```python
from build123d import *

# Parameters (mm, degrees)
SKETCH1_W            = 59.589999946
SKETCH1_H            = 23.283333334
BOSS_EXTRUDE1_DEPTH  = 2.929999982
SKETCH2_W            = 2.929999982
SKETCH2_H            = 11.641666667
CUT_EXTRUDE1_DEPTH   = 3.929999982
BOSS_EXTRUDE3_DEPTH  = 2.93
FILLET1_R            = 0.2
SKETCH5_R            = 0.25
CUT_EXTRUDE3_DEPTH   = 3.93
FILLET2_R            = 0.5
FILLET1_OF_MIRROR1_R = 0.2
FILLET2_OF_MIRROR1_R = 0.5
SKETCH3_W            = 44.45
SKETCH3_H            = 16.933333334
CUT_EXTRUDE2_DEPTH   = 1


with BuildPart() as part:
    # Sketch1 → Boss-Extrude1 (new body)
    with BuildSketch(Plane.XY):
        Rectangle(SKETCH1_W, SKETCH1_H)
    extrude(amount=BOSS_EXTRUDE1_DEPTH)

    # Sketch2 → Cut-Extrude1 (cut, through all)
    with BuildSketch(Plane.XY.offset(2.929999982)):
        with Locations((-26.864999991, -5.820833334)):
            Rectangle(SKETCH2_W, SKETCH2_H)
    cut_extrude1 = extrude(amount=-CUT_EXTRUDE1_DEPTH, mode=Mode.SUBTRACT)

    # Sketch4 → Boss-Extrude3 (add)
    with BuildSketch(Plane.XY.offset(2.929999982)):
        Polygon((-27.329999982, -8.711666685), (-28.329999982, -8.711666685), (-28.329999982, -10.711666685), (-27.329999982, -9.711666685), align=None)
    boss_extrude3 = extrude(amount=-BOSS_EXTRUDE3_DEPTH)

    # Fillet1
    fillet1_edges = [part.edges().sort_by_distance(p)[0] for p in [
        (-27.329999982, -8.711666685, 1.464999982),
        (-28.329999982, -10.711666685, 1.464999982),
        (-27.329999982, -9.711666685, 1.464999982),
    ]]
    fillet(fillet1_edges, radius=FILLET1_R)

    # Sketch5 → Cut-Extrude3 (cut, through all)
    with BuildSketch(Plane.XY.offset(2.929999982)):
        with Locations((-28.329999982, 0)):
            Circle(SKETCH5_R)
    cut_extrude3 = extrude(amount=-CUT_EXTRUDE3_DEPTH, mode=Mode.SUBTRACT)

    # Fillet2
    fillet2_edges = [part.edges().sort_by_distance(p)[0] for p in [
        (-28.079999982, 0, 1.464999991),
        (-28.329999982, -0.25, 1.464999991),
    ]]
    fillet(fillet2_edges, radius=FILLET2_R)

    # Mirror1: Cut-Extrude1, Boss-Extrude3, Cut-Extrude3 across plane
    add(cut_extrude1.mirror(Plane(origin=(0, 0, 0), x_dir=(0, 0, 1), z_dir=(1, 0, 0))), mode=Mode.SUBTRACT)
    add(boss_extrude3.mirror(Plane(origin=(0, 0, 0), x_dir=(0, 0, 1), z_dir=(1, 0, 0))))
    add(cut_extrude3.mirror(Plane(origin=(0, 0, 0), x_dir=(0, 0, 1), z_dir=(1, 0, 0))), mode=Mode.SUBTRACT)

    # Fillet1 of Mirror1
    fillet1_of_mirror1_edges = [part.edges().sort_by_distance(p)[0] for p in [
        (27.329999982, -8.711666685, 1.464999982),
        (28.329999982, -10.711666685, 1.464999982),
        (27.329999982, -9.711666685, 1.464999982),
    ]]
    fillet(fillet1_of_mirror1_edges, radius=FILLET1_OF_MIRROR1_R)

    # Fillet2 of Mirror1
    fillet2_of_mirror1_edges = [part.edges().sort_by_distance(p)[0] for p in [
        (28.079999982, 0, 1.464999991),
        (28.329999982, -0.25, 1.464999991),
    ]]
    fillet(fillet2_of_mirror1_edges, radius=FILLET2_OF_MIRROR1_R)

    # Sketch3 → Cut-Extrude2 (cut)
    with BuildSketch(Plane.XY.offset(2.929999982)):
        Rectangle(SKETCH3_W, SKETCH3_H)
    extrude(amount=-CUT_EXTRUDE2_DEPTH, mode=Mode.SUBTRACT)


solid = part.part
```
Design review of the part built by this model. Coordinates are the model's own, in mm. A direction names the side the tool comes from. Give positions to 0.01 mm unless a question says otherwise; leave off trailing zeros. Order: outer loops, then holes, each group sorted by start corner. A loop starts at its lowest first (then second) coordinate and runs counter-clockwise, first axis right, second up. Notation, with made-up numbers: (64.5, 0.5) -> (97.5, 0.5) arc R28 ccw to (97.5, 30.5) -> close; hole circle Ø2 at (-32.75, 52.5). An arc over 180 degrees is marked (long way). Write item = value, one per line. Start each with the question number.
(1) Mouldability with a two-part tool opening along X and no side actions: class faces 4 (the face through (0, 9, 2.93)), 5 (the face through (-29.795, 0, 1)), 6 (the face through (-22.225, -0.1, 2.4)) as +X half, -X half, draft (parallel to the pull), parting line (faces both ways), or undercut.
(2) For faces 1 (the face through (-0.3, 8.467, 2.4)), 2 (the face through (25.4, -6, 1)), 3 (the face through (-27, 0, 1)), list the 3-axis set-ups (+Z, -Z, +X, -X, +Y, -Y) from which the entire face can be reached by the end or side of a thin tool; tool diameter is ignored.
(3) We need section A-A on y = -4.5. Write out the cut boundary in (x, z) (3 decimals), plus the area to 3 significant figures.
(4) We need section B-B on x = 4. Write out the cut boundary in (y, z).
(5) To check wall thickness, follow line 1 along X through (y, z) = (-8, 2.15) (3 decimals); line 2 along X through (y, z) = (-3.75, 0.95) (3 decimals); line 3 along Y through (x, z) = (13, 2.4). State the ranges of each line that lie inside material, in increasing order.
(6) We need section D-D on y = 7.5. Write out the cut boundary in (x, z) (3 decimals), plus the area to 3 significant figures.
(7) For pin 1 (3 mm diameter, centred on x = -23, y = -3.5, fed in from -Z), flat-tipped, find the tip position at first contact; note if it passes through.
Numbers:
q1.face_4 = draft
q1.face_5 = -X half
q1.face_6 = undercut
q2.face_1 = +Z
q2.face_2 = +Z, -Z, -Y
q2.face_3 = +Z, -Z
q3.outline = (-29.795, 0) -> (-28.33, 0) -> (-28.33, 2.93) -> (-29.795, 2.93) -> close; (-25.4, 0) -> (25.4, 0) -> (25.4, 2.93) -> (22.225, 2.93) -> (22.225, 1.93) -> (-22.225, 1.93) -> (-22.225, 2.93) -> (-25.4, 2.93) -> close; (28.33, 0) -> (29.795, 0) -> (29.795, 2.93) -> (28.33, 2.93) -> close
q3.area = 113 mm^2
q4.outline = (-11.64, 0) -> (11.64, 0) -> (11.64, 2.93) -> (8.47, 2.93) -> (8.47, 1.93) -> (-8.47, 1.93) -> (-8.47, 2.93) -> (-11.64, 2.93) -> close
q5.line_1 = -29.795 to -28.33, -25.4 to -22.225, 22.225 to 25.4, 28.33 to 29.795
q5.line_2 = -29.795 to -28.33, -25.4 to 25.4, 28.33 to 29.795
q5.line_3 = -11.64 to -8.47, 8.47 to 11.64
q6.outline = (-29.795, 0) -> (29.795, 0) -> (29.795, 2.93) -> (22.225, 2.93) -> (22.225, 1.93) -> (-22.225, 1.93) -> (-22.225, 2.93) -> (-29.795, 2.93) -> close
q6.area = 130 mm^2
q7.pin_1 = 0
